Autodesk Inventor part; units mm, degrees
ref_plane "YZ Plane" through (0, 0, 0) normal (1, 0, 0) x (0, 1, 0)
ref_plane "XZ Plane" through (0, 0, 0) normal (0, 1, 0) x (-1, 0, 0)
ref_plane "XY Plane" through (0, 0, 0) normal (0, 0, 1) x (1, 0, 0)
ref_plane "Work Plane1" through (0, 0, 10) normal (0, 0, 1) x (1, 0, 0)
sketch "Sketch1" plane through (0, 0, 10) normal (0, 0, 1) x (1, 0, 0)
  line L0 (-4.0299, -0.3538) -> (-2.2322, 1.4439) construction
  arc A0 (-1.4439, 2.2322) -> (-2.2322, 1.4439) centre (-0.9299, 0.9299) ccw construction
  line L1 (-1.4439, 2.2322) -> (0.3538, 4.0299) construction
  line L2 (-37.8299, 42.8299) -> (-37.8299, 37.8299) construction
  line L3 (-37.8299, 37.8299) -> (-42.9208, 37.8299) construction
  line L4 (-37.8299, 42.2137) -> (-37.8299, 45.8299) construction
  line L5 (-37.8299, 45.8299) -> (-4.0299, 45.8299) construction
  line L6 (-4.0299, 45.8299) -> (-4.0299, 42.2137) construction
  line L7 (-4.0299, 4.0299) -> (0.3538, 4.0299)
  circle A1 centre (-20.9299, 20.9299) radius 17.5
  line L8 (-20.9299, 58.9723) -> (17.1124, 20.9299) construction
  line L9 (17.1124, 20.9299) -> (-20.9299, -17.1124) construction
  line L10 (-20.9299, -17.1124) -> (-58.9723, 20.9299) construction
  line L11 (-58.9723, 20.9299) -> (-20.9299, 58.9723) construction
  line L12 (-20.9299, 58.9723) -> (-20.9299, -17.1124) construction
  line L13 (17.1124, 20.9299) -> (-58.9723, 20.9299) construction
  line L14 (-20.9299, 58.9723) -> (32.8701, 58.9723) construction
  line L15 (-43.4299, 43.4299) -> (1.5701, 43.4299) construction
  line L16 (1.5701, 43.4299) -> (1.5701, -1.5701) construction
  line L17 (1.5701, -1.5701) -> (-43.4299, -1.5701) construction
  line L18 (-43.4299, -1.5701) -> (-43.4299, 43.4299) construction
  line L19 (-43.4299, 43.4299) -> (1.5701, -1.5701) construction
  line L20 (1.5701, 43.4299) -> (-43.4299, -1.5701) construction
  line L21 (-43.4299, 5.3876) -> (-43.4299, 36.4723)
  line L22 (-43.4299, 36.4723) -> (-36.4723, 43.4299)
  line L23 (-36.4723, 43.4299) -> (-5.3876, 43.4299)
  line L24 (-5.3876, 43.4299) -> (1.5701, 36.4723)
  line L25 (1.5701, 36.4723) -> (1.5701, 5.3876)
  line L26 (1.5701, 5.3876) -> (-5.3876, -1.5701)
  line L27 (-5.3876, -1.5701) -> (-36.4723, -1.5701)
  line L28 (-36.4723, -1.5701) -> (-43.4299, 5.3876)
  line L29 (-4.0299, 42.2137) -> (-37.8299, 42.2137)
  line L30 (-4.0299, -0.3538) -> (-4.0299, 4.0299)
  circle A2 centre (-20.9299, 20.9299) radius 1.5
  line L31 (-10.9299, 10.9299) -> (-30.9299, 10.9299) construction
  line L32 (-30.9299, 10.9299) -> (-30.9299, 30.9299) construction
  line L33 (-30.9299, 30.9299) -> (-10.9299, 30.9299) construction
  line L34 (-10.9299, 30.9299) -> (-10.9299, 10.9299) construction
  line L35 (-10.9299, 10.9299) -> (-30.9299, 30.9299) construction
  line L36 (-30.9299, 10.9299) -> (-10.9299, 30.9299) construction
  circle A3 centre (-30.9299, 30.9299) radius 1.4
  circle A4 centre (-30.9299, 10.9299) radius 1.4
  circle A5 centre (-10.9299, 10.9299) radius 1.4
  line L37 (-45.8299, 37.8299) -> (-42.0723, 37.8299) construction
  line L38 (-42.1723, 37.7299) -> (-45.8299, 37.7299)
  line L39 (-45.8299, 37.7299) -> (-45.8299, 4.1299)
  line L40 (-45.8299, 4.1299) -> (-42.1723, 4.1299)
  line L41 (-42.1723, 4.1299) -> (-42.1723, 37.7299)
  line L42 (-45.8299, 4.0299) -> (-42.0723, 4.0299) construction
  line L43 (-45.8299, 37.8299) -> (-42.0723, 37.8299)
  line L44 (-37.7299, 45.8299) -> (-4.1299, 45.8299)
  line L45 (-4.1299, 45.8299) -> (-4.1299, 42.1723)
  line L46 (-4.1299, 42.1723) -> (-37.7299, 42.1723)
  line L47 (-37.7299, 42.1723) -> (-37.7299, 45.8299)
  line L48 (0.4701, 37.8299) -> (0.4701, 4.0299) construction
  line L49 (0.4701, 4.0299) -> (3.9701, 4.0299) construction
  line L50 (3.9701, 37.8299) -> (3.9701, 4.0299) construction
  line L51 (0.4701, 37.8299) -> (3.9701, 37.8299) construction
  line L52 (-45.8299, -3.9701) -> (-4.0299, -3.9701) construction
  line L53 (0.3124, 37.7299) -> (3.9701, 37.7299)
  line L54 (3.9701, 37.7299) -> (3.9701, 4.1299)
  line L55 (3.9701, 4.1299) -> (0.3124, 4.1299)
  line L56 (0.3124, 4.1299) -> (0.3124, 37.7299)
  line L57 (-4.1713, -0.3538) -> (-37.7299, -0.3538)
  line L58 (-37.7299, -0.3538) -> (-37.7299, -3.9701)
  line L59 (-37.7299, -3.9701) -> (-4.1713, -3.9701)
  line L60 (-4.1713, -3.9701) -> (-4.1713, -0.3538)
  point P0 (-37.8299, 4.0299)
  dimension "d18" = 53.8
  dimension "d19" = 45
  dimension "d20" = 53.8
  dimension "d21" = 45
  dimension "d22" = 45
  dimension "d30" = 20
  dimension "d31" = 20
  dimension "d32" = 2.8
  dimension "d33" = 2.8
  dimension "d34" = 2.8
  dimension "d35" = 3
  dimension "d36" = 0.1
  dimension "d37" = 0.1
  dimension "d38" = 0.1
  dimension "d39" = 0.1
extrude "Extrusion1" add sketch "Sketch1" along normal blind 5 contours L30 L26 L57 L28 L41 L22 L46 L24 L56 L7 | L7 L26 L30 | L56 L24 L25 L26 | L26 L25 L24 L53 L54 L55 | L60 L59 L58 L57 L28 L27 L26 | L26 L27 L28 L57 | L46 L22 L29 L24 | L24 L29 L45 | L40 L39 L38 L22 L21 L28 | L28 L21 L22 L41 | L29 L22 L23 L24 | L24 L23 L22 L29 L47 L44 L45 | L47 L29 L22 | A1
properties part number "20_Cube_Insert_Kinematic_Mirrormount_base"
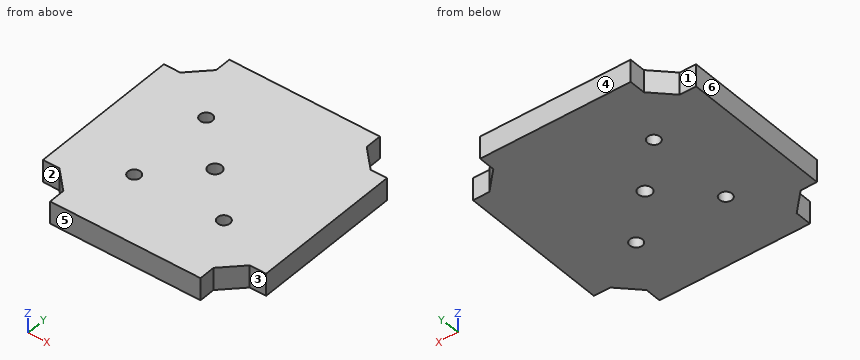
Could you check a few things on this model? Use its own coordinates, in mm. Face numbers are marked on the shaded views. A direction names the side the tool comes from. Coordinates: 2 decimals unless noted, no trailing zeros. Write each loop counter-clockwise with the first axis right and the second up, starting at its lowest first coordinate (ties: lowest second). Pieces come first, ordered by that corner, then holes. Notation, with made-up numbers: (26, 4) - (48, 4) arc R21 ccw to (48, 31) - close; hole circle Ø6 at (26.5, 51.5). An arc over 180 degrees is marked (long way). Write item = value, one per line.
1) Suppose I cut it at D-D on y = 40. Please give me the cut outline in (x, z).
Result set:
outline = (-39.9, 10) - (-1.96, 10) - (-1.96, 15) - (-39.9, 15) - close
2) Suppose I cut it at B-B on z = 12.9. Please give me the cut outline in (x, y).
Result set:
outline = (-45.83, 4.13) - (-42.17, 4.13) - (-37.69, -0.35) - (-37.73, -0.35) - (-37.73, -3.97) - (-4.17, -3.97) - (-4.17, -0.35) - (0.31, 4.13) - (3.97, 4.13) - (3.97, 37.73) - (0.31, 37.73) - (-4.13, 42.17) - (-4.13, 45.83) - (-37.73, 45.83) - (-37.73, 42.17) - (-42.17, 37.73) - (-45.83, 37.73) - close; hole circle Ø2.8 at (-30.93, 10.93); hole circle Ø2.8 at (-30.93, 30.93); hole circle Ø3 at (-20.93, 20.93); hole circle Ø2.8 at (-10.93, 10.93)
3) Will these pins go through, and if not, where does the flat tip stop? pin 1 Ø3 at (y, z) = (44.5, 12.5) entering from -X; pin 2 Ø1.1 at (x, z) = (-44, 11.5) entering from -Y; pin 3 Ø1.8 at (x, z) = (-44.5, 13) entering from +Y.
Result set:
pin_1 = -37.73
pin_2 = 4.13
pin_3 = 37.73
4) Please list where these lines run through material, in increasing order: line 1 (Y direction, x = -30.5, z = 11.65); line 2 (Y direction, x = -43, z = 14.75); line 3 (Y direction, x = -39.5, z = 13.55). Write a range as [from, to].
Result set:
line_1 = [-3.97, 9.6], [12.26, 29.6], [32.26, 45.83]
line_2 = [4.13, 37.73]
line_3 = [1.46, 40.4]
5) For the marked faces 1, 2 and 3, which set-ups out of +Z, -Z, +X, -X, +Y, -Y let a thin tool reach every point of the face, with its end or its side?
Result set:
face_1 = +Z, -Z, -X, +Y
face_2 = +Z, -Z, -X, -Y
face_3 = +Z, -Z, +X, -Y
6) Suppose I cut it at A-A on x = -20.5. Please give me the cut outline in (y, z).
Result set:
outline = (-3.97, 10) - (19.49, 10) - (19.49, 15) - (-3.97, 15) - close; (22.37, 10) - (45.83, 10) - (45.83, 15) - (22.37, 15) - close
7) Suppose I cut it at C-C on x = -11.5. Please give me the cut outline in (y, z), plus the area to 3 significant figures.
Result set:
outline = (-3.97, 10) - (9.65, 10) - (9.65, 15) - (-3.97, 15) - close; (12.21, 10) - (45.83, 10) - (45.83, 15) - (12.21, 15) - close
area = 236 mm2
8) We'd pull the mould along Y, two halves only. Please class the marked faces 4, 5 and 6: +Y half, -Y half, draft (parallel to the pull), parting line (faces both ways), or undercut.
Result set:
face_4 = +Y half
face_5 = -Y half
face_6 = draft
